from build123d import *

# Parameters (mm, degrees)
SKETCH_W         = 65
SKETCH_H         = 36
PAD_DEPTH        = 2
SKETCH001_W      = 65
SKETCH001_H      = 36
SKETCH001_W_2    = 61
SKETCH001_H_2    = 32
PAD001_DEPTH     = 10
SKETCH002_R      = 3.5
PAD002_DEPTH     = 5
HOLE_D           = 5
HOLE_CSINK_D     = 5.2
HOLE_CSINK_ANGLE = 8
SKETCH003_W      = 8
SKETCH003_H      = 14
POCKET_DEPTH     = 12.001
SKETCH004_W      = 11
SKETCH004_H      = 17
SKETCH004_W_2    = 8
SKETCH004_H_2    = 14
PAD003_DEPTH     = 10
FILLET_R         = 2


with BuildPart() as part:
    # Sketch → Pad (new body)
    with BuildSketch(Plane.XY):
        Rectangle(SKETCH_W, SKETCH_H)
    extrude(amount=PAD_DEPTH)

    # Sketch001 → Pad001 (join)
    with BuildSketch(Plane.XY.offset(2)):
        Rectangle(SKETCH001_W, SKETCH001_H)
        Rectangle(SKETCH001_W_2, SKETCH001_H_2, mode=Mode.SUBTRACT)
    extrude(amount=PAD001_DEPTH)

    # Sketch002 → Pad002 (join)
    with BuildSketch(Plane.XY):
        with Locations((-26.5, 12.1)):
            Circle(SKETCH002_R)
        with Locations((-21.1, -12.2)):
            Circle(SKETCH002_R)
        with Locations((23.7, 11.9)):
            Circle(SKETCH002_R)
        with Locations((18.1, -12.2)):
            Circle(SKETCH002_R)
    extrude(amount=PAD002_DEPTH)

    # Hole (through all)
    with Locations(Plane(origin=(0, 0, 0), x_dir=(1, 0, 0), z_dir=(0, 0, -1))):
        with Locations((-26.5, -12.1), (-21.1, 12.2), (23.7, -11.9), (18.1, 12.2)):
            CounterSinkHole(HOLE_D / 2, HOLE_CSINK_D / 2, counter_sink_angle=HOLE_CSINK_ANGLE)

    # Sketch003 → Pocket (cut, through all)
    with BuildSketch(Plane.XY):
        with Locations((-18.5, 0.4)):
            Rectangle(SKETCH003_W, SKETCH003_H)
    extrude(amount=POCKET_DEPTH, mode=Mode.SUBTRACT)

    # Sketch004 → Pad003 (join)
    with BuildSketch(Plane.XY.offset(2)):
        with Locations((-18.5, 0.4)):
            Rectangle(SKETCH004_W, SKETCH004_H)
        with Locations((-18.5, 0.4)):
            Rectangle(SKETCH004_W_2, SKETCH004_H_2, mode=Mode.SUBTRACT)
    extrude(amount=PAD003_DEPTH)

    # Fillet
    fillet_edges = [part.edges().sort_by_distance(p)[0] for p in [
        (-32.5, -18, 7),
        (-30.5, -16, 7),
        (-32.5, 18, 7),
        (-30.5, 16, 7),
        (32.5, -18, 7),
        (30.5, -16, 7),
        (30.5, 16, 7),
        (32.5, 18, 7),
        (-13, -8.1, 7),
        (-24, -8.1, 7),
        (-22.5, -6.6, 7),
        (-14.5, -6.6, 7),
        (-24, 8.9, 7),
        (-22.5, 7.4, 7),
        (-13, 8.9, 7),
        (-14.5, 7.4, 7),
    ]]
    fillet(fillet_edges, radius=FILLET_R)


solid = part.part
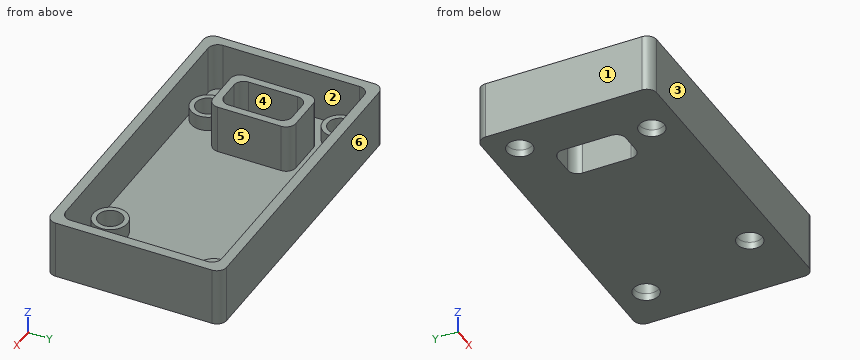
CAD build for the part. Positions are in the model's coordinates, mm. Face numbers are marked on the shaded views. A direction names the side the tool comes from. Coordinates: 2 decimals unless noted, no trailing zeros. Write each loop counter-clockwise with the first axis right and the second up, starting at its lowest first coordinate (ties: lowest second). Pieces come first, ordered by that corner, then holes. Notation, with made-up numbers: M 59.25,-23.5 L 67.25,-23.5 A16 ccw 67.25,-9.5 Z; hole C 70,46 d6. An arc over 180 degrees is marked long. Return JSON: item names as keys, results as strings.
Item 1: Two-plate mould, pull along Y, no slides. Class the marked faces 1, 2 and 3: +Y half, -Y half, draft (parallel to the pull), parting line (faces both ways), or undercut.
Findings below:
{"face 1": "draft", "face 2": "undercut", "face 3": "-Y half"}
Item 2: Which spindle directions (+Z, -Z, +X, -X, +Y, -Y) get a long thin tool onto all of the face, cutting with end or side? Do the marked faces 4, 5 and 6. Say none if no direction does.
Findings below:
{"face 4": "+Z, -Z", "face 5": "+Z", "face 6": "+Z, -Z, +X, -X, +Y"}
Item 3: Slice it at D-D, the plane x = 8. Write the cut outline in (y, z).
Findings below:
{"outline": "M -18,0 L 18,0 L 18,12 L 16,12 L 16,2 L -16,2 L -16,12 L -18,12 Z"}
Item 4: Probe line 1 (X direction, y = 5, z = 6); line 2 (Y direction, x = 23.7, z = 2.25); line 3 (Y direction, x = -26.5, z = 4.5). List the from-to ranges inside material, lowest first. Write a range as from..to.
Findings below:
{"line 1": "x = -32.5..-30.5, -24..-22.5, -14.5..-13, 30.5..32.5", "line 2": "y = -18..-16, 8.4..9.4, 14.4..15.4, 16..18", "line 3": "y = -18..-16, 8.6..9.6, 14.6..15.6, 16..18"}
Item 5: Slice it at C-C, the plane x = 23.7. Write the cut outline in (y, z), and give its area (3 significant figures).
Findings below:
{"outline": "M -18,0 L 9.3,0 L 9.4,1.43 L 9.4,5 L 8.4,5 L 8.4,2 L -16,2 L -16,12 L -18,12 Z; M 14.4,1.43 L 14.5,0 L 18,0 L 18,12 L 16,12 L 16,2 L 15.4,2 L 15.4,5 L 14.4,5 Z", "area": "108 mm2"}
Item 6: Slice it at B-B, the plane y = -12.2. Write the cut outline in (x, z).
Findings below:
{"outline": "M -32.5,0 L -23.7,0 L -23.6,1.43 L -23.6,5 L -24.6,5 L -24.6,2 L -30.5,2 L -30.5,12 L -32.5,12 Z; M -18.6,1.43 L -18.5,0 L 15.5,0 L 15.6,1.43 L 15.6,5 L 14.6,5 L 14.6,2 L -17.6,2 L -17.6,5 L -18.6,5 Z; M 20.6,1.43 L 20.7,0 L 32.5,0 L 32.5,12 L 30.5,12 L 30.5,2 L 21.6,2 L 21.6,5 L 20.6,5 Z"}
Item 7: Slice it at A-A, the plane z = 9. State how many separate pieces and enclosed holes the cut face has, and give its area (3 significant figures).
Findings below:
{"separate pieces": "2", "enclosed holes": "2", "area": "463 mm2"}
Item 8: Drop flat-ended pins along their axis: pin 1 Ø2 at (x, y) = (-22, -12) entering from +Z; pin 2 Ø9.5 at (x, y) = (10.5, 5.5) entering from +Z; pin 3 Ø2 at (x, y) = (19, -10.5) entering from +Z. Give the stop position or say it passes through.
Findings below:
{"pin 1": "passes through", "pin 2": "stops at z = 2", "pin 3": "stops at z = 5"}
